```python
from build123d import *

# Parameters (mm, degrees)
SKETCH1_W               = 253
SKETCH1_H               = 50
BOSS_EXTRUDE1_DEPTH     = 17.5
SKETCH2_W               = 47
SKETCH2_H               = 22
CUT_EXTRUDE1_DEPTH      = 10
SKETCH4_W               = 22
SKETCH4_H               = 31
CUT_EXTRUDE2_DEPTH      = 15
MIRROR2_COPY_1_SKETCH_W = 47
MIRROR2_COPY_1_SKETCH_H = 22
MIRROR2_COPY_1_DEPTH    = 10
MIRROR2_COPY_2_SKETCH_W = 22
MIRROR2_COPY_2_SKETCH_H = 31
MIRROR2_COPY_2_DEPTH    = 15


with BuildPart() as part:
    # Sketch1 → Boss-Extrude1 (new body)
    with BuildSketch(Plane(origin=(0, 0, 0), x_dir=(1, 0, 0), z_dir=(0, 1, 0))):
        with Locations((126.5, -10)):
            Rectangle(SKETCH1_W, SKETCH1_H)
    extrude(amount=BOSS_EXTRUDE1_DEPTH)

    # Sketch2 → Cut-Extrude1 (cut)
    with BuildSketch(Plane(origin=(0, 17.5, 0), x_dir=(1, 0, 0), z_dir=(0, 1, 0))):
        with Locations((26.5, -15)):
            Rectangle(SKETCH2_W, SKETCH2_H)
    cut_extrude1 = extrude(amount=-CUT_EXTRUDE1_DEPTH, mode=Mode.SUBTRACT)

    # Sketch4 → Cut-Extrude2 (cut)
    with BuildSketch(Plane(origin=(0, 17.5, 0), x_dir=(1, 0, 0), z_dir=(0, 1, 0))):
        with Locations((26.5, -19.5)):
            Rectangle(SKETCH4_W, SKETCH4_H)
    cut_extrude2 = extrude(amount=-CUT_EXTRUDE2_DEPTH, mode=Mode.SUBTRACT)

    # Mirror1: Cut-Extrude1, Cut-Extrude2 across plane
    add(cut_extrude1.mirror(Plane.ZY.offset(-51.5)), mode=Mode.SUBTRACT)
    add(cut_extrude2.mirror(Plane.ZY.offset(-51.5)), mode=Mode.SUBTRACT)

    # Mirror2: Cut-Extrude1, Cut-Extrude2 across plane
    add(cut_extrude1.mirror(Plane.ZY.offset(-101.5)), mode=Mode.SUBTRACT)
    add(cut_extrude2.mirror(Plane.ZY.offset(-101.5)), mode=Mode.SUBTRACT)

    # Mirror2 copy 1 sketch → Mirror2 copy 1 (cut)
    with BuildSketch(Plane(origin=(100, 17.5, 0), x_dir=(1, 0, 0), z_dir=(0, 1, 0))):
        with Locations((26.5, -15)):
            Rectangle(MIRROR2_COPY_1_SKETCH_W, MIRROR2_COPY_1_SKETCH_H)
    extrude(amount=-MIRROR2_COPY_1_DEPTH, mode=Mode.SUBTRACT)

    # Mirror2 copy 2 sketch → Mirror2 copy 2 (cut)
    with BuildSketch(Plane(origin=(100, 17.5, 0), x_dir=(1, 0, 0), z_dir=(0, 1, 0))):
        with Locations((26.5, -19.5)):
            Rectangle(MIRROR2_COPY_2_SKETCH_W, MIRROR2_COPY_2_SKETCH_H)
    extrude(amount=-MIRROR2_COPY_2_DEPTH, mode=Mode.SUBTRACT)

    # Mirror3: Cut-Extrude1, Cut-Extrude2 across plane
    add(cut_extrude1.mirror(Plane.ZY.offset(-126.5)), mode=Mode.SUBTRACT)
    add(cut_extrude2.mirror(Plane.ZY.offset(-126.5)), mode=Mode.SUBTRACT)


solid = part.part
```
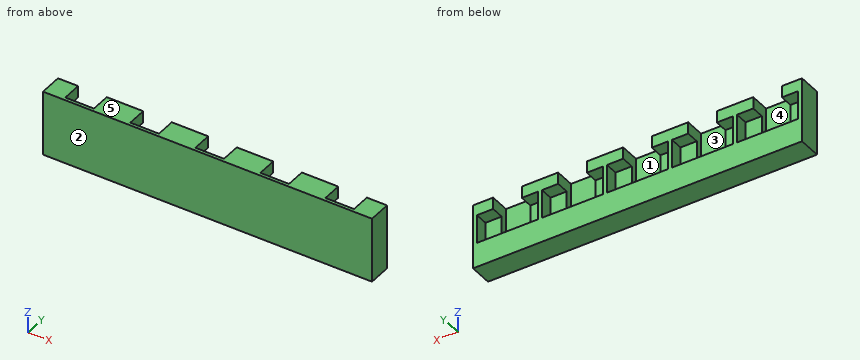
Work out the finished part from the listing and answer in its coordinate system (mm). Face numbers are marked on the shaded views. A direction names the side the tool comes from. Give positions to 0.01 mm unless a question says otherwise; leave off trailing zeros. Loops run counter-clockwise (first coordinate to the right, second up) from the corner with the lowest first, then second, coordinate; pieces in that order, holes last. Notation, with made-up numbers: (18.5, 21.25) -> (36.5, 21.25) arc R19 cw to (36.5, 55.25) -> close; hole circle Ø11 at (0, 26). An arc over 180 degrees is marked (long way). Put each result on its own line as item: value. Start each with the question number.
Item 1: Find the intervals of material crossed by L1, parallel to X at y = 14.25, z = 27; L2, parallel to X at y = 10, z = 12.5; L3, parallel to Z at x = 110.5, y = 14, in increasing order. Write a range as [from, to].
Item 2: Which of the six approach directions +Z, -Z, +X, -X, +Y, -Y give full straight-line access (tool end or side, diameter ignored) to the marked faces 4 and 5?
Item 3: The part is cut by section B-B (z = 28.5). Give the vertices of the cut face in (x, y), then the cut area to 3 significant figures.
Item 4: The part is cut by section C-C (y = 5.25). Give the vertices of the cut face in (x, z), then the cut area to 3 significant figures.
Item 5: The mould has two halves that part along X. Classify the marked faces 1, 2 and 3: released by +X, released by -X, zero draft, split by the parting line, or undercut.
Item 6: The part is cut by section A-A (x = 162). Give the vertices of the cut face in (y, z).
Item 7: Each of these flat-tipped pins is pushed along its axis until it touches: P1, Ø6.5, axis at x = 29.5, z = 20.5, coming from the +Y side; P2, Ø6, axis at x = 58.5, z = 9.5, coming from the +Y side. Where does it stop, or does it pass through?
Answers below:
1. L1: [0, 15.5], [37.5, 65.5], [87.5, 115.5], [137.5, 165.5], [187.5, 215.5], [237.5, 253]
1. L2: [0, 3], [50, 53], [100, 103], [150, 153], [200, 203], [250, 253]
1. L3: [-15, 4], [26, 35]
2. face 4: +Z, +Y
2. face 5: +Z, +X, -X, +Y, -Y
3. outline: (0, 0) -> (253, 0) -> (253, 17.5) -> (237.5, 17.5) -> (237.5, 2.5) -> (215.5, 2.5) -> (215.5, 17.5) -> (187.5, 17.5) -> (187.5, 2.5) -> (165.5, 2.5) -> (165.5, 17.5) -> (137.5, 17.5) -> (137.5, 2.5) -> (115.5, 2.5) -> (115.5, 17.5) -> (87.5, 17.5) -> (87.5, 2.5) -> (65.5, 2.5) -> (65.5, 17.5) -> (37.5, 17.5) -> (37.5, 2.5) -> (15.5, 2.5) -> (15.5, 17.5) -> (0, 17.5) -> close
3. area: 2,780 mm2
4. outline: (0, -15) -> (253, -15) -> (253, 35) -> (237.5, 35) -> (237.5, 4) -> (215.5, 4) -> (215.5, 35) -> (187.5, 35) -> (187.5, 4) -> (165.5, 4) -> (165.5, 35) -> (137.5, 35) -> (137.5, 4) -> (115.5, 4) -> (115.5, 35) -> (87.5, 35) -> (87.5, 4) -> (65.5, 4) -> (65.5, 35) -> (37.5, 35) -> (37.5, 4) -> (15.5, 4) -> (15.5, 35) -> (0, 35) -> close
4. area: 9,240 mm2
5. face 1: undercut
5. face 2: zero draft
5. face 3: undercut
6. outline: (0, -15) -> (17.5, -15) -> (17.5, 4) -> (7.5, 4) -> (7.5, 26) -> (17.5, 26) -> (17.5, 35) -> (0, 35) -> close
7. P1: y = 2.5
7. P2: y = 7.5
